Build history of the part. All positions in model axes, mm. Face numbers are marked on the shaded views. A direction names the side the tool comes from. Give positions to 0.01 mm unless a question says otherwise; leave off trailing zeros. Write each loop counter-clockwise with the first axis right and the second up, starting at its lowest first coordinate (ties: lowest second). Pieces come first, ordered by that corner, then holes. Notation, with made-up numbers: (-26, 0) -> (29, 0) arc R15 cw to (29, 29) -> close; hole circle Ø4 at (56.25, 83). An arc over 180 degrees is marked (long way). One line per question, with ' | ' between items. Start each with the question number.
(1) Tool access for the marked faces 1 and 2: list every direction of +Z, -Z, +X, -X, +Y, -Y with a clear straight run to the whole face (end or side of a thin tool).
(2) Band-saw the part on B-B, the plane z = -7.75. Give the cut face in (x, y).
(3) Drill centre lines: probe 1 along X at (y, z) = (46, -21); probe 2 along Z at (x, y) = (-148.25, 52.5); probe 3 along Z at (x, y) = (-100, 9). Where is each one in solid material? Low to high. Write a range as from..to.
(4) Pull direction X, two halves, no side cores. Call the marked faces 3, 4 and 5: released by +X, released by -X, zero draft, split by the parting line, or undercut.
(5) Pin check, flat tips, straight feed: P1, Ø5.5, axis at x = -3, z = -4, coming from the -Y side; P2, Ø4, axis at x = -1.5, z = -4, coming from the +Y side; P3, Ø1, axis at x = -24, y = 45.5, coming from the -Z side. Stop position of each tip, or through.
(6) Band-saw the part on D-D, the plane x = -134.5. Give the cut face in (y, z).
(7) Band-saw the part on C-C, the plane y = 61. Give the cut face in (x, z).
(8) Band-saw the part on A-A, the plane y = 52.5. Give the cut face in (x, z), and give its area (3 significant figures).
from build123d import *

# Parameters (mm, degrees)
SKETCH1_W           = 150
SKETCH1_H           = 80
BOSS_EXTRUDE1_DEPTH = 5
SKETCH2_W           = 5
SKETCH2_H           = 25
BOSS_EXTRUDE2_DEPTH = 25
SKETCH3_R           = 5
CUT_EXTRUDE1_DEPTH  = 151
FILLET1_R           = 10


with BuildPart() as part:
    # Sketch1 → Boss-Extrude1 (new body)
    with BuildSketch(Plane.XY):
        with Locations((-75, 40)):
            Rectangle(SKETCH1_W, SKETCH1_H)
    extrude(amount=BOSS_EXTRUDE1_DEPTH)

    # Sketch2 → Boss-Extrude2 (add)
    with BuildSketch(Plane(origin=(0, 0, 0), x_dir=(-1, 0, 0), z_dir=(0, 0, -1))):
        with Locations((2.5, 52.5)):
            Rectangle(SKETCH2_W, SKETCH2_H)
        with Locations((147.5, 52.5)):
            Rectangle(SKETCH2_W, SKETCH2_H)
    extrude(amount=BOSS_EXTRUDE2_DEPTH)

    # Sketch3 → Cut-Extrude1 (cut, through all)
    with BuildSketch(Plane(origin=(0, 0, 0), x_dir=(0, 0, -1), z_dir=(1, 0, 0))):
        with Locations(Location((15, 52.5, 0), (0, 0, 90))):  # turned: the seam where the file's is
            Circle(SKETCH3_R)
    extrude(amount=-CUT_EXTRUDE1_DEPTH, mode=Mode.SUBTRACT)

    # Fillet1
    fillet1_edges = [part.edges().sort_by_distance(p)[0] for p in [
        (-2.5, 40, -25),
        (-2.5, 65, -25),
        (-147.5, 65, -25),
        (-147.5, 40, -25),
    ]]
    fillet(fillet1_edges, radius=FILLET1_R)


solid = part.part
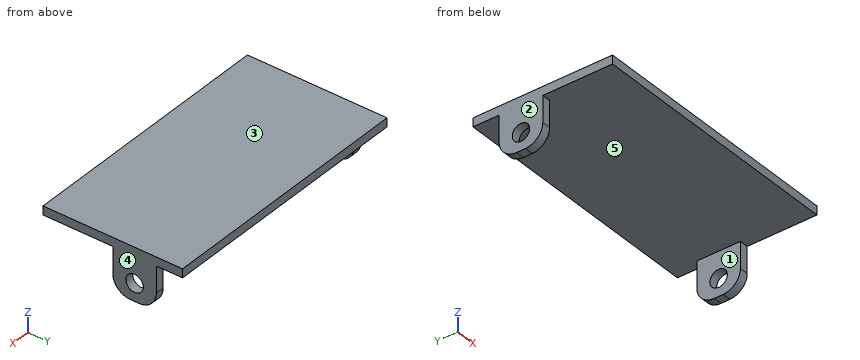
Results:
1) face 1: -Z, +Y, -Y | face 2: +Z, -Z, -X, +Y, -Y
2) outline: (-150, 40) -> (-145, 40) -> (-145, 65) -> (-150, 65) -> close; (-5, 40) -> (0, 40) -> (0, 65) -> (-5, 65) -> close
3) probe 1: x = -150..-145, -5..0 | probe 2: z = -25..-20, -10..5 | probe 3: z = 0..5
4) face 3: zero draft | face 4: released by +X | face 5: undercut
5) P1: stops at y = 40 | P2: stops at y = 65 | P3: stops at z = 0
6) outline: (0, 0) -> (80, 0) -> (80, 5) -> (0, 5) -> close
7) outline: (-150, -23) -> (-145, -23) -> (-145, 0) -> (-5, 0) -> (-5, -23) -> (0, -23) -> (0, 5) -> (-150, 5) -> close
8) outline: (-150, -25) -> (-145, -25) -> (-145, -20) -> (-150, -20) -> close; (-150, -10) -> (-145, -10) -> (-145, 0) -> (-5, 0) -> (-5, -10) -> (0, -10) -> (0, 5) -> (-150, 5) -> close; (-5, -25) -> (0, -25) -> (0, -20) -> (-5, -20) -> close | area: 900 mm²
